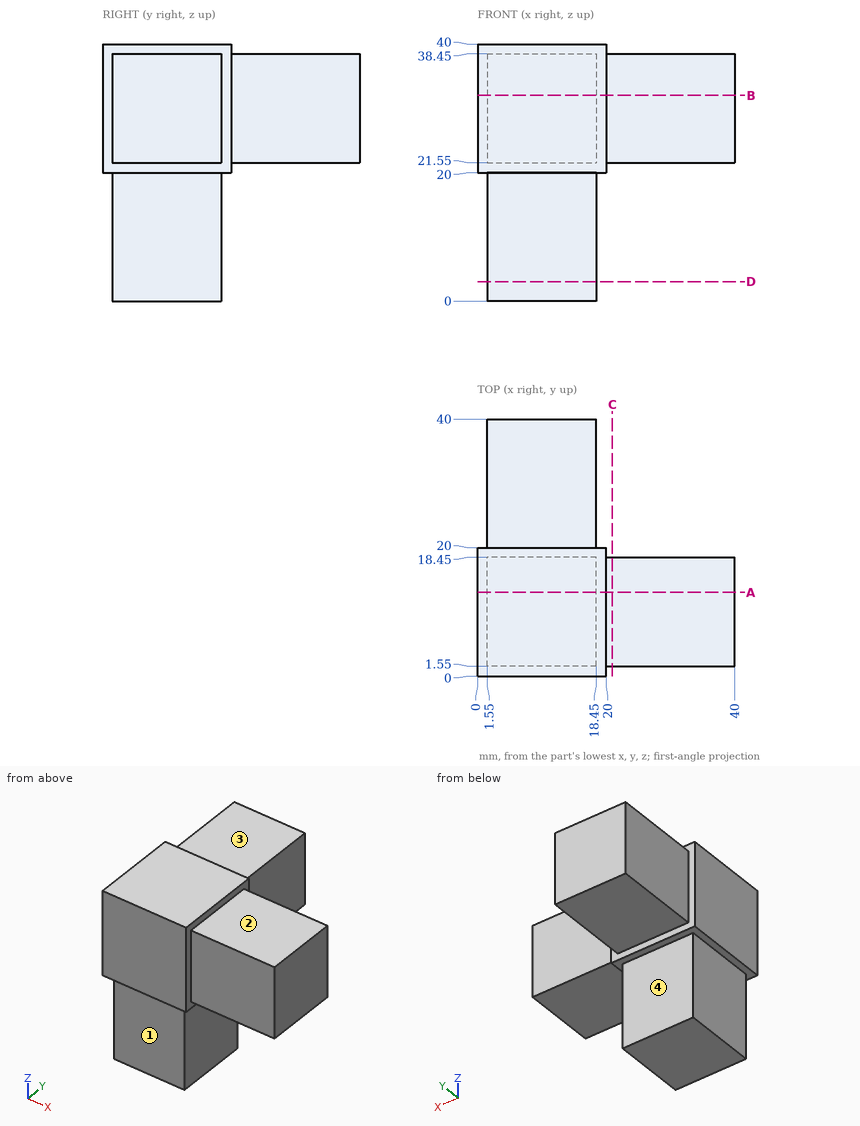
Answer from the drawing. Dimensions are ordinates in mm from the lowest x, y and z of the part. A direction names the side the tool comes from. Give positions to 0.01 mm unless a question says otherwise; leave off trailing zeros. Loops run counter-clockwise (first coordinate to the right, second up) from the corner with the lowest first, then second, coordinate; pieces in that order, holes last. Notation, with made-up numbers: (86.5, -38.75) -> (145.5, -38.75) arc R20 cw to (145.5, -28.75) -> close; hole circle Ø6 at (76, -18). An arc over 180 degrees is marked (long way). Use a Markdown table: item, result.
Q1. Each of these flat-tipped pins is pushed along its axis until it touches: pin 1 (5 mm diameter, centred on y = 11, z = 7.5, fed in from -X); pin 2 (8.5 mm diameter, centred on x = 8.5, y = 31, fed in from +Z); pin 3 (2 mm diameter, centred on x = 31.5, y = 18, fed in from -Z). Where does it stop, or does it pass through?
Solved:
| item | result |
|---|---|
| pin 1 | stops at x = 1.55 |
| pin 2 | stops at z = 38.45 |
| pin 3 | stops at z = 21.55 |
Q2. Section D-D, the plane z = 3 is taken. Determine the outline of the cut face in (x, y), then the cut area to 3 significant figures.
Solved:
| item | result |
|---|---|
| outline | (1.55, 1.55) -> (18.45, 1.55) -> (18.45, 18.45) -> (1.55, 18.45) -> close |
| area | 286 mm^2 |
Q3. A tool of negligible diameter and unlimited length cuts with its end or side. For the marked faces 1, 2, 3 and 4, from which of +Z, -Z, +X, -X, +Y, -Y can it reach the whole face along a straight path? Write none if from no direction.
Solved:
| item | result |
|---|---|
| face 1 | -Z, +X, -X, -Y |
| face 2 | +Z, +X, +Y, -Y |
| face 3 | +Z, +X, -X, +Y |
| face 4 | -Z, +X, -X, +Y |
Q4. Section C-C, the plane x = 21 is taken. Determine the outline of the cut face in (y, z).
Solved:
| item | result |
|---|---|
| outline | (1.55, 21.55) -> (18.45, 21.55) -> (18.45, 38.45) -> (1.55, 38.45) -> close |
Q5. Section A-A, the plane y = 13 is taken. Determine the outline of the cut face in (x, z).
Solved:
| item | result |
|---|---|
| outline | (0, 20) -> (1.55, 20) -> (1.55, 0) -> (18.45, 0) -> (18.45, 20) -> (20, 20) -> (20, 21.55) -> (40, 21.55) -> (40, 38.45) -> (20, 38.45) -> (20, 40) -> (0, 40) -> close |
Q6. Section B-B, the plane z = 32 is taken. Determine the outline of the cut face in (x, y).
Solved:
| item | result |
|---|---|
| outline | (0, 0) -> (20, 0) -> (20, 1.55) -> (40, 1.55) -> (40, 18.45) -> (20, 18.45) -> (20, 20) -> (18.45, 20) -> (18.45, 40) -> (1.55, 40) -> (1.55, 20) -> (0, 20) -> close |
Q7. Find the intervals of material crossed by line 1 along Z through (x, y) = (32.5, 11); line 2 along Y through (x, z) = (17, 13.5), in increasing order.
Solved:
| item | result |
|---|---|
| line 1 | z = 21.55 to 38.45 |
| line 2 | y = 1.55 to 18.45 |
